The listing builds one solid part. Answer for the finished solid, in the listing's coordinates (mm). Face numbers are marked on the shaded views. A direction names the side the tool comes from. Coordinates: 2 decimals unless noted, no trailing zeros. Order: outer loops, then holes, each group sorted by start corner. A loop starts at its lowest first (then second) coordinate and runs counter-clockwise, first axis right, second up. Notation, with made-up numbers: (-24.75, -9) -> (-0.75, -9) arc R25 ccw to (-0.75, 4) -> close; hole circle Ø11 at (77.25, 75). An arc over 180 degrees is marked (long way). Answer in a Markdown table with one row per item.
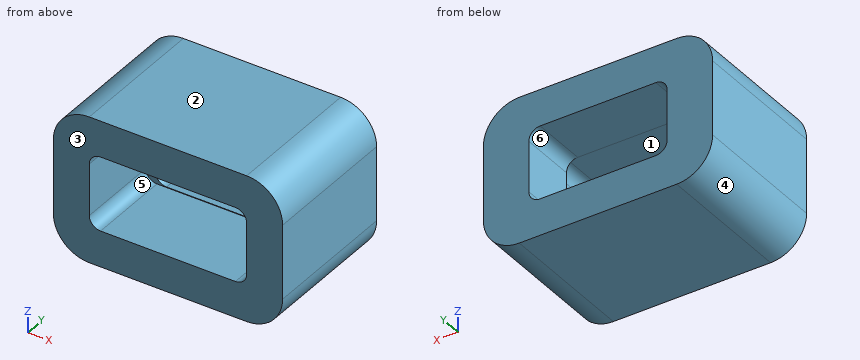
```python
from build123d import *

# Parameters (mm, degrees)
SKETCH058_W     = 20.4
SKETCH058_H     = 13
PAD032_DEPTH    = 12.5
SKETCH059_W     = 14
SKETCH059_H     = 6.6
POCKET027_DEPTH = 7.5
SKETCH060_W     = 12.3
SKETCH060_H     = 6.5
POCKET028_DEPTH = 5
FILLET027_R     = 1
FILLET028_R     = 3.2


with BuildPart() as part:
    # Sketch058 → Pad032 (new body)
    with BuildSketch(Plane.XZ):
        with Locations((10.2, 6.5)):
            Rectangle(SKETCH058_W, SKETCH058_H)
    extrude(amount=PAD032_DEPTH)

    # Sketch059 (on Face6 of Pad032) → Pocket027 (cut)
    with BuildSketch(Plane.XZ.offset(12.5)):
        with Locations((10.2, 6.5)):
            Rectangle(SKETCH059_W, SKETCH059_H)
    extrude(amount=-POCKET027_DEPTH, mode=Mode.SUBTRACT)

    # Sketch060 (on Face4 of Pocket027) → Pocket028 (cut)
    with BuildSketch(Plane(origin=(0, 0, 0), x_dir=(1, 0, 0), z_dir=(0, 1, 0))):
        with Locations((10.2, -6.5)):
            Rectangle(SKETCH060_W, SKETCH060_H)
    extrude(amount=-POCKET028_DEPTH, mode=Mode.SUBTRACT)

    # Fillet027
    fillet027_edges = [part.edges().sort_by_distance(p)[0] for p in [
        (16.35, -2.5, 9.75),
        (4.05, -2.5, 9.75),
        (4.05, -2.5, 3.25),
        (16.35, -2.5, 3.25),
        (17.2, -8.75, 9.8),
        (17.2, -8.75, 3.2),
        (3.2, -8.75, 3.2),
        (3.2, -8.75, 9.8),
    ]]
    fillet(fillet027_edges, radius=FILLET027_R)

    # Fillet028
    fillet028_edges = [part.edges().sort_by_distance(p)[0] for p in [
        (0, -6.25, 13),
        (0, -6.25, 0),
        (20.4, -6.25, 13),
        (20.4, -6.25, 0),
    ]]
    fillet(fillet028_edges, radius=FILLET028_R)


solid = part.part
```
(1) Which of the six approach directions +Z, -Z, +X, -X, +Y, -Y give full straight-line access (tool end or side, diameter ignored) to the marked faces 4, 5 and 6?
Check values:
| item | result |
|---|---|
| face 4 | -Z, -X, +Y, -Y |
| face 5 | -Y |
| face 6 | +Y, -Y |
(2) Find the intervals of material crossed by line 1 along Z through (x, y) = (6.75, -2); line 2 along X through (y, z) = (-10.75, 7.5); line 3 along X through (y, z) = (-4.25, 7.75), in increasing order. Write a range as from..to.
Check values:
| item | result |
|---|---|
| line 1 | 0..3.25, 9.75..13 |
| line 2 | 0..3.2, 17.2..20.4 |
| line 3 | 0..4.05, 16.35..20.4 |
(3) A cutting plane is placed at B-B, the plane y = -9.5. Determine the outline of the cut face in (x, z).
Check values:
| item | result |
|---|---|
| outline | (0, 3.2) arc R3.2 ccw to (3.2, 0) -> (17.2, 0) arc R3.2 ccw to (20.4, 3.2) -> (20.4, 9.8) arc R3.2 ccw to (17.2, 13) -> (3.2, 13) arc R3.2 ccw to (0, 9.8) -> close; hole (3.2, 4.2) arc R1 ccw to (4.2, 3.2) -> (16.2, 3.2) arc R1 ccw to (17.2, 4.2) -> (17.2, 8.8) arc R1 ccw to (16.2, 9.8) -> (4.2, 9.8) arc R1 ccw to (3.2, 8.8) -> close |
(4) A cutting plane is placed at C-C, the plane x = 8.5. Determine the outline of the cut face in (y, z), then the cut area to 3 significant figures.
Check values:
| item | result |
|---|---|
| outline | (-12.5, 0) -> (0, 0) -> (0, 3.25) -> (-5, 3.25) -> (-5, 3.2) -> (-12.5, 3.2) -> close; (-12.5, 9.8) -> (-5, 9.8) -> (-5, 9.75) -> (0, 9.75) -> (0, 13) -> (-12.5, 13) -> close |
| area | 80.5 mm² |
(5) A cutting plane is placed at D-D, the plane x = 3.5. Determine the outline of the cut face in (y, z).
Check values:
| item | result |
|---|---|
| outline | (-12.5, 0) -> (0, 0) -> (0, 13) -> (-12.5, 13) -> (-12.5, 9.51) -> (-5, 9.51) -> (-5, 3.49) -> (-12.5, 3.49) -> close |
(6) A flat-ended cylindrical pin translates along its axis: pin 1 (5.5 mm diameter, centred on x = 12, z = 7.5, fed in from -Y). Find the tip coordinate at first contact, or state that the pin passes through.
Check values:
| item | result |
|---|---|
| pin 1 | y = -12.5 |
(7) For a pull along Z with two mould halves and no side action, classify the marked faces 1, 2 and 3 as released by +Z, released by -Z, zero draft, split by the parting line, or undercut.
Check values:
| item | result |
|---|---|
| face 1 | undercut |
| face 2 | released by +Z |
| face 3 | zero draft |
(8) A cutting plane is placed at A-A, the plane z = 7.75. Determine the outline of the cut face in (x, y).
Check values:
| item | result |
|---|---|
| outline | (0, -12.5) -> (3.2, -12.5) -> (3.2, -5) -> (4.05, -5) -> (4.05, 0) -> (0, 0) -> close; (16.35, -5) -> (17.2, -5) -> (17.2, -12.5) -> (20.4, -12.5) -> (20.4, 0) -> (16.35, 0) -> close |
